Work out the finished part from the listing and answer in its coordinate system (mm). Give positions to 0.01 mm unless a question says otherwise; leave off trailing zeros. Loops run counter-clockwise (first coordinate to the right, second up) from the corner with the lowest first, then second, coordinate; pieces in that order, holes last. Notation, with made-up numbers: (-40, -5) - (-33, -5) arc R20 ccw to (-33, 22) - close; hole circle Ø7 at (6, 73). An arc over 180 degrees is marked (long way). Use CSV: the item, a comma, the result in double quotes.
from build123d import *

# Parameters (mm, degrees)
F1_DEPTH = 4
F2_COUNT = 8
F4_R     = 5.5
F5_DEPTH = 4


with BuildPart() as f1:
    # F0 (on Top) → F1 (new body)
    with BuildSketch(Plane.XY):
        with BuildLine():
            Line((0, 22.28635), (0, 26.502684))
            ThreePointArc((0, 26.502684), (-9.016314, 19.375069), (0, 12.247453))
            ThreePointArc((0, 12.247453), (10.336376, 6.123727), (0, 0))
            Line((0, 0), (0, -6.289178))
            ThreePointArc((0, -6.289178), (13.747998, 5.231544), (0, 16.752267))
            ThreePointArc((0, 16.752267), (-6.104504, 19.519308), (0, 22.28635))
        make_face()
    extrude(amount=F1_DEPTH)


with BuildPart() as f2_1:
    # F2: instance of F1
    add(f1.part.rotate(Axis((0, -6.289178, 2), (0, 0, 1)), 1 * 360 / F2_COUNT))


with BuildPart() as f2_2:
    # F2: instance of F1
    add(f1.part.rotate(Axis((0, -6.289178, 2), (0, 0, 1)), 2 * 360 / F2_COUNT))


with BuildPart() as f2_3:
    # F2: instance of F1
    add(f1.part.rotate(Axis((0, -6.289178, 2), (0, 0, 1)), 3 * 360 / F2_COUNT))


with BuildPart() as f2_4:
    # F2: instance of F1
    add(f1.part.rotate(Axis((0, -6.289178, 2), (0, 0, 1)), 4 * 360 / F2_COUNT))


with BuildPart() as f2_5:
    # F2: instance of F1
    add(f1.part.rotate(Axis((0, -6.289178, 2), (0, 0, 1)), 5 * 360 / F2_COUNT))


with BuildPart() as f2_6:
    # F2: instance of F1
    add(f1.part.rotate(Axis((0, -6.289178, 2), (0, 0, 1)), 6 * 360 / F2_COUNT))


with BuildPart() as f2_7:
    # F2: instance of F1
    add(f1.part.rotate(Axis((0, -6.289178, 2), (0, 0, 1)), 7 * 360 / F2_COUNT))


with BuildPart() as f2_6_1:
    add(f2_6.part)

    # F3: union F2_7, F2_5, F2_2, F2_1, F2_4, F2_3, F1
    add(f2_7.part)
    add(f2_5.part)
    add(f2_2.part)
    add(f2_1.part)
    add(f2_4.part)
    add(f2_3.part)
    add(f1.part)

    # F4 (on face) → F5 (cut)
    with BuildSketch(Plane.XY.offset(4)):
        with Locations((0, -7.159515)):
            Circle(F4_R)
    extrude(amount=-F5_DEPTH, mode=Mode.SUBTRACT)


solid = f2_6_1.part
Item 1: A cutting plane is placed at A-A on y = -31. Determine the outline of the cut face in (x, z), and give its area (3 significant figures).
Determined:
outline,"(-21.94, 0) - (-11.97, 0) - (-11.97, 4) - (-21.94, 4) - close; (5.94, 0) - (8.95, 0) - (8.95, 4) - (5.94, 4) - close"
area,"51.9 mm²"
Item 2: Given P1, Ø2, axis at x = 31, z = 2, coming from the -Y side; P2, Ø1.5, axis at x = 4, z = 1, coming from the -Y side; P3, Ø1.5, axis at x = -16.5, z = 1, coming from the -Y side, each flat-ended and moving along its own axis, determine where each tip first touches the part or whether it passes through.
Determined:
P1,"stops at y = -6.29"
P2,"stops at y = -39.11"
P3,"stops at y = -32.96"
Item 3: A cutting plane is placed at B-B on x = 12. Determine the outline of the cut face in (y, z), and give its area (3 significant figures).
Determined:
outline,"(-26.31, 0) - (-21.62, 0) - (-21.62, 4) - (-26.31, 4) - close; (-20.03, 0) - (-16.61, 0) - (-16.61, 4) - (-20.03, 4) - close; (-11.04, 0) - (-6.81, 0) - (-6.81, 4) - (-11.04, 4) - close; (-0.92, 0) - (18.45, 0) - (18.45, 4) - (-0.92, 4) - close"
area,"127 mm²"
Item 4: The mould has two halves that part along X. Classify faces 1 (the cylindrical face through (12.4, -26.1, 2)), 2 (the flat face through (21.68, 15.39, 1.97)), 3 (the cylindrical face through (-5.221, -29.072, 1.972)), 4 (the flat face through (-31, -6.289, 2)): pulls with the +X half, pulls with the -X half, needs draft (parallel to the pull), parting line crosses it, or undercut.
Determined:
face 1,"undercut"
face 2,"pulls with the +X half"
face 3,"undercut"
face 4,"needs draft"
Item 5: Find the intervals of material crossed by line 1 (X direction, y = 15, z = 3.85); line 2 (Y direction, x = -17.5, z = 3.75); line 3 (Y direction, x = -6.5, z = 2.9), in increasing order.
Determined:
line 1,"x = -25.25 to -21.29, -7.57 to 8.49, 9.89 to 13.1, 19.97 to 21.29"
line 2,"y = -32.94 to -29.8, -21.61 to -15.6, -9.79 to -4.36, 1.85 to 7.51"
line 3,"y = -28.63 to -24.94, -12.47 to -1.7, 0.78 to 6.33, 11.84 to 24.9"
Item 6: A cutting plane is placed at C-C on x = -15. Determine the outline of the cut face in (y, z).
Determined:
outline,"(-32.69, 0) - (-29.6, 0) - (-29.6, 4) - (-32.69, 4) - close; (-22.91, 0) - (-18.52, 0) - (-18.52, 4) - (-22.91, 4) - close; (-6.87, 0) - (-2.61, 0) - (-2.61, 4) - (-6.87, 4) - close; (3.55, 0) - (11.55, 0) - (11.55, 4) - (3.55, 4) - close"
Item 7: A cutting plane is placed at D-D on z = 0.85. State how many separate pieces and enclosed holes the cut face has, and give its area (3 significant figures).
Determined:
separate pieces,"1"
enclosed holes,"9"
area,"1,380 mm²"
